from build123d import *

# Parameters (mm, degrees)
F0_W           = 62.8
F0_H           = 62.8
F0_W_2         = 51
F0_H_2         = 51
F0_W_3         = 45
F0_H_3         = 45
F1_DEPTH       = 4
F2_DEPTH       = 3
F4_D           = 2.4384
F4_DEPTH       = 20
F4_CSINK_D     = 5.0038
F4_CSINK_ANGLE = 82
F4_TIP         = 0.7325692667
F5_D           = 2.4384
F5_DEPTH       = 20
F5_START       = 3
F5_TIP         = 0.7325692667
F7_DEPTH       = 4.001
F8_SIZE        = 5


with BuildPart() as f1:
    # F0 (on Top) → F1 (new body)
    with BuildSketch(Plane.XY):
        Rectangle(F0_W, F0_H)
        Rectangle(F0_W_2, F0_H_2, mode=Mode.SUBTRACT)
        Rectangle(F0_W_2, F0_H_2)
        Rectangle(F0_W_3, F0_H_3, mode=Mode.SUBTRACT)
    extrude(amount=F1_DEPTH)

    # F0 (on Top) → F2 (cut)
    with BuildSketch(Plane.XY):
        Rectangle(F0_W_2, F0_H_2)
        Rectangle(F0_W_3, F0_H_3, mode=Mode.SUBTRACT)
    extrude(amount=F2_DEPTH, mode=Mode.SUBTRACT)

    # F4
    with Locations(Plane.XY.offset(4)):
        with Locations((-17.4625, -28.49), (-28.49, -17.4625), (-28.49, 17.4625), (-17.4625, 28.49), (17.4625, 28.49), (28.49, 17.4625), (28.49, -17.4625), (17.4625, -28.49)):
            CounterSinkHole(F4_D / 2, F4_CSINK_D / 2, depth=F4_DEPTH, counter_sink_angle=F4_CSINK_ANGLE)
            with Locations((0, 0, -(F4_DEPTH + F4_TIP / 2))):  # 118° drill point
                Cone(0, F4_D / 2, F4_TIP, mode=Mode.SUBTRACT)

    # F5
    # its depths count from where the whole tool has entered the part; down to there all is cleared
    with Locations(Plane(origin=(0, 0, 0), x_dir=(1, 0, 0), z_dir=(0, 0, -1)).offset(-F5_START)):
        with Locations((-25.5, -25.5), (25.5, -25.5), (-25.5, 25.5), (25.5, 25.5)):
            Hole(F5_D / 2, depth=F5_DEPTH)
            with Locations((0, 0, -(F5_DEPTH + F5_TIP / 2))):  # 118° drill point
                Cone(0, F5_D / 2, F5_TIP, mode=Mode.SUBTRACT)

    # F6 (on face) → F7 (cut, through all)
    with BuildSketch(Plane.XY.offset(4)):
        with BuildLine():
            Line((-21.2808, 22.5), (-24.2808, 25.5))
            ThreePointArc((-24.2808, 25.5), (-24.6378954124, 24.6378954124), (-25.5, 24.2808))
            Line((-25.5, 24.2808), (-22.5, 21.2808))
            Line((-22.5, 21.2808), (-22.5, 22.5))
            Line((-22.5, 22.5), (-21.2808, 22.5))
        make_face()
        with BuildLine():
            Line((22.5, 21.2808), (25.5, 24.2808))
            ThreePointArc((25.5, 24.2808), (24.6378954124, 24.6378954124), (24.2808, 25.5))
            Line((24.2808, 25.5), (21.2808, 22.5))
            Line((21.2808, 22.5), (22.5, 22.5))
            Line((22.5, 22.5), (22.5, 21.2808))
        make_face()
        with BuildLine():
            ThreePointArc((-25.5, -24.2808), (-24.6378954124, -24.6378954124), (-24.2808, -25.5))
            Line((-24.2808, -25.5), (-21.2808, -22.5))
            Line((-21.2808, -22.5), (-22.5, -22.5))
            Line((-22.5, -22.5), (-22.5, -21.2808))
            Line((-22.5, -21.2808), (-25.5, -24.2808))
        make_face()
        with BuildLine():
            ThreePointArc((24.2808, -25.5), (24.6378954124, -24.6378954124), (25.5, -24.2808))
            Line((25.5, -24.2808), (22.5, -21.2808))
            Line((22.5, -21.2808), (22.5, -22.5))
            Line((22.5, -22.5), (21.2808, -22.5))
            Line((21.2808, -22.5), (24.2808, -25.5))
        make_face()
    extrude(amount=-F7_DEPTH, mode=Mode.SUBTRACT)

    # F8
    f8_edges = [f1.edges().sort_by_distance(p)[0] for p in [
        (31.4, -31.4, 2),
        (-31.4, -31.4, 2),
        (-31.4, 31.4, 2),
        (31.4, 31.4, 2),
    ]]
    chamfer(f8_edges, length=F8_SIZE)


solid = f1.part
Could you check a few things on this model? Use its own coordinates, in mm. A direction names the side the tool comes from. Give positions to 0.01 mm unless a question says otherwise; leave off trailing zeros. Write each loop counter-clockwise with the first axis right and the second up, starting at its lowest first coordinate (ties: lowest second). Pieces come first, ordered by that corner, then holes. Notation, with made-up numbers: (-23.75, 79) -> (1.25, 79) arc R18 ccw to (1.25, 99) -> close; hole circle Ø7 at (82, 40). An arc over 180 degrees is marked (long way). Write each question's results on one line, items separated by ' | '. Start each with the question number.
Q1. We'd pull the mould along Y, two halves only. Please class faces 4 (the face through (0, -31.4, 2)), 5 (the face through (16.81, 29.52, 1.24)), 6 (the face through (-24, 0, 3)), 7 (the face through (-31.4, 0, 2)): +Y half, -Y half, draft (parallel to the pull), parting line (faces both ways), or undercut.
Q2. Suppose I cut it at A-A, the plane x = 14. List the corners of the cut face in (y, z) for me.
Q3. Suppose I cut it at C-C, the plane x = 28.49. List the corners of the cut face in (y, z) for me.
Q4. I'm going to push a flat-ended pin straight in: pin 1 Ø0.9 at (x, y) = (23.5, 10.5) entering from -Z. Where does the tip first touch, or does it pass through?
Q5. I need wall thicknesses on probe 1 along Y at (x, z) = (-17.5, 0.5); probe 2 along Y at (x, z) = (-21, 0.6); probe 3 along Y at (x, z) = (28, 1.85). Which ranges of each line are inside material? Lowest first, please.
Q6. Which directions (+Z, -Z, +X, -X, +Y, -Y) give clear straight access to the entire face, cutting with the end or side of a thin tool? Please do faces 1 (the face through (28.9, -28.9, 2)), 2 (the face through (-24.02, 22.8, 3.51)), 3 (the face through (0, -25.5, 1)).
Outcome:
1) face 4: -Y half | face 5: undercut | face 6: undercut | face 7: draft
2) outline: (-31.4, 0) -> (-25.5, 0) -> (-25.5, 3) -> (-22.5, 3) -> (-22.5, 4) -> (-31.4, 4) -> close; (22.5, 3) -> (25.5, 3) -> (25.5, 0) -> (31.4, 0) -> (31.4, 4) -> (22.5, 4) -> close
3) outline: (-29.31, 0) -> (-18.68, 0) -> (-18.68, 2.52) -> (-19.96, 4) -> (-29.31, 4) -> close; (-16.24, 0) -> (16.24, 0) -> (16.24, 2.52) -> (14.96, 4) -> (-14.96, 4) -> (-16.24, 2.52) -> close; (18.68, 0) -> (29.31, 0) -> (29.31, 4) -> (19.96, 4) -> (18.68, 2.52) -> close
4) pin 1: z = 3
5) probe 1: -31.4 to -29.71, -27.27 to -25.5, 25.5 to 27.27, 29.71 to 31.4 | probe 2: -31.4 to -25.5, 25.5 to 31.4 | probe 3: -29.8 to -18.58, -16.35 to 16.35, 18.58 to 29.8
6) face 1: +Z, -Z, +X, -Y | face 2: +Z, -Z | face 3: -Z
